Can you work these out from the model? Positions are in its coordinate system, mm. Coordinates: 2 decimals unless noted, no trailing zeros. Loops run counter-clockwise (first coordinate to the right, second up) from the corner with the lowest first, then second, coordinate; pieces in that order, holes last. Notation, with made-up numbers: M 80,65.5 L 84,65.5 A26 cw 84,95.5 Z; hole C 28.5,-23.75 d8. An arc over 180 degrees is marked long. Answer as a JSON object with one key per item and string values. Group by question number.
Item 1: Suppose I cut it at C-C (y = 70). Write out the boundary of the cut face in (x, z), then the cut area to 3 significant figures.
Item 2: I'm going to push flat-ended pins straight in: pin 1 Ø4 at (x, y) = (8.5, -30.5) entering from -Z; pin 2 Ø3 at (x, z) = (10.5, 98.5) entering from -Y; pin 3 Ø24 at (y, z) = (0, 0) entering from -X; pin 4 Ø6 at (x, z) = (5, -45.5) entering from -Y. Where does each tip first touch, or does it pass through?
Item 3: Suppose I cut it at B-B (x = 10). Count the separate pieces of the cut face and the enclosed holes in it, then the cut area to 3 significant figures.
Item 4: Suppose I cut it at D-D (z = -91.5). Write out the boundary of the cut face in (x, y), then the cut area to 3 significant figures.
Item 5: Suppose I cut it at A-A (z = 0). Write out the boundary of the cut face in (x, y), then the cut area to 3 significant figures.
Item 6: If I drill on line 1 (X direction, y = -48, z = -13.5); line 2 (Y direction, x = 5.5, z = -0.5); line 3 (Y direction, x = 3.5, z = -98), over which ranges is the centre line in solid material (lowest first)?
Autodesk Inventor part; units mm, degrees
ref_plane "YZ Plane" through (0, 0, 0) normal (1, 0, 0) x (0, 1, 0)
ref_plane "XZ Plane" through (0, 0, 0) normal (0, 1, 0) x (-1, 0, 0)
ref_plane "XY Plane" through (0, 0, 0) normal (0, 0, 1) x (1, 0, 0)
sketch "Sketch1" plane through (0, 0, 0) normal (1, 0, 0) x (0, 1, 0)
  circle A0 centre (0, 0) radius 125
  dimension "d0" = 250
extrude "Extrusion1" add sketch "Sketch1" along normal blind 3
sketch "Sketch2" plane through (3, 0, 0) normal (1, 0, 0) x (0, 0, -1)
  circle A0 centre (0, 0) radius 15
  line L0 (0, 0) -> (0, 70) construction
  circle A1 centre (0, 70) radius 7.5
  circle A2 centre (-49.4975, 49.4975) radius 7.5
  circle A3 centre (-70, 0) radius 7.5
  circle A4 centre (-49.4975, -49.4975) radius 7.5
  circle A5 centre (0, -70) radius 7.5
  circle A6 centre (49.4975, -49.4975) radius 7.5
  circle A7 centre (70, 0) radius 7.5
  circle A8 centre (49.4975, 49.4975) radius 7.5
  line L1 (0, 0) -> (92.388, 38.2683) construction
  line L2 (0, 0) -> (100, 0) construction
  circle A9 centre (92.388, 38.2683) radius 7.5
  circle A10 centre (38.2683, 92.388) radius 7.5
  circle A11 centre (-38.2683, 92.388) radius 7.5
  circle A12 centre (-92.388, 38.2683) radius 7.5
  circle A13 centre (-92.388, -38.2683) radius 7.5
  circle A14 centre (-38.2683, -92.388) radius 7.5
  circle A15 centre (38.2683, -92.388) radius 7.5
  circle A16 centre (92.388, -38.2683) radius 7.5
  dimension "d3" = 30
  dimension "d4" = 70
  dimension "d5" = 15
  dimension "d8" = 360
  dimension "d10" = 100
  dimension "d11" = 22.5
  dimension "d12" = 15
  dimension "d15" = 360
extrude "Extrusion2" add sketch "Sketch2" along normal blind 10 contours A1 | A2 | A3 | A4 | A5 | A6 | A7 | A8 | A9 | A10 | A11 | A12 | A13 | A14 | A15 | A16
ref_plane "Work Plane1" through (8, -49.4975, 49.4975) normal (1, 0, 0) x (0, 0, -1)
mirror "Mirror1" about plane through (8, -49.4975, 49.4975) normal (1, 0, 0) of "Extrusion1"
sketch "Sketch3" plane through (16, 0, 0) normal (1, 0, 0) x (0, 0, -1)
  circle A0 centre (0, 0) radius 15
  dimension "d20" = 30
extrude "Extrusion3" cut sketch "Sketch3" against normal through all
properties part number "Base Plate"
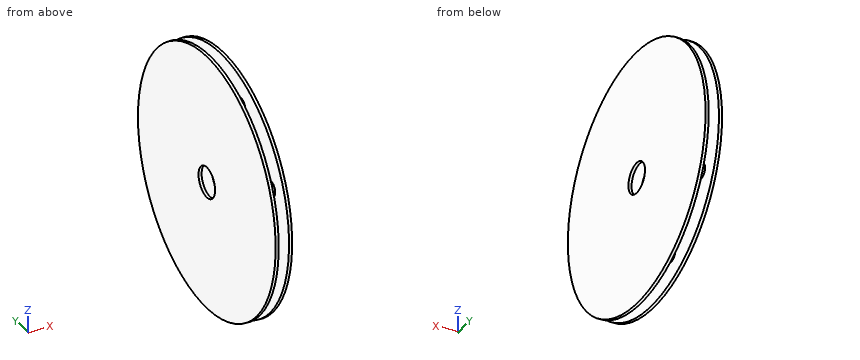
From the geometry:
{
 "1": {"outline": "M 0,-103.56 L 3,-103.56 L 3,-7.5 L 13,-7.5 L 13,-103.56 L 16,-103.56 L 16,103.56 L 13,103.56 L 13,7.5 L 3,7.5 L 3,103.56 L 0,103.56 Z", "area": "1,390 mm2"},
 "2": {"pin 1": "z = -97.18", "pin 2": "y = -44.18", "pin 3": "through", "pin 4": "y = -117.27"},
 "3": {"separate pieces": "16", "enclosed holes": "0", "area": "2,830 mm2"},
 "4": {"outline": "M 0,-85.16 L 3,-85.16 L 3,-45.72 L 13,-45.72 L 13,-85.16 L 16,-85.16 L 16,85.16 L 13,85.16 L 13,45.72 L 3,45.72 L 3,85.16 L 0,85.16 Z; hole M 3,-30.82 L 13,-30.82 L 13,30.82 L 3,30.82 Z", "area": "1,320 mm2"},
 "5": {"outline": "M 0,-125 L 3,-125 L 3,-77.5 L 13,-77.5 L 13,-125 L 16,-125 L 16,-15 L 13,-15 L 13,-62.5 L 3,-62.5 L 3,-15 L 0,-15 Z; M 0,15 L 3,15 L 3,62.5 L 13,62.5 L 13,15 L 16,15 L 16,125 L 13,125 L 13,77.5 L 3,77.5 L 3,125 L 0,125 Z", "area": "1,620 mm2"},
 "6": {"line 1": "0 to 3, 13 to 16", "line 2": "-77.48 to -62.52, 62.52 to 77.48", "line 3": "-43.24 to -33.29, 33.29 to 43.24"}
}
